Input: part model. Units: mm. Frame: model coordinates. Round coordinates to 2 decimals unless told otherwise and drop trailing zeros. Order: outer loops, then holes, each group sorted by start corner. A loop starts at its lowest first (then second) coordinate and runs counter-clockwise, first axis right, second up. Notation, with made-up numbers: (76, -13) -> (90, -13) arc R34 ccw to (90, 21) -> close; hole circle Ø3 at (14.25, -8.5). An arc over 180 degrees is marked (long way). Use a Markdown table: item, result.
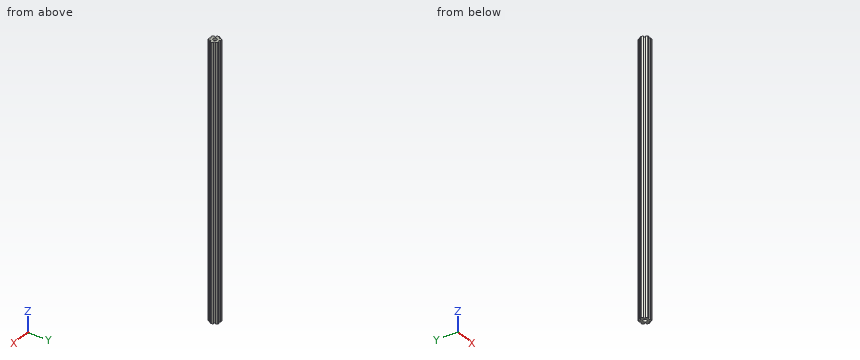
from build123d import *

# Parameters (mm, degrees)
BOSS_EXTRUDE1_DEPTH     = 355.6
SKETCH2_R               = 1.27
SKETCH2_R_2             = 2.54
CUT_EXTRUDE1_DEPTH      = 356.6
FILLET1_R               = 0.508
F_1_4_20_TAPPED_HOLE3_D = 5.1054


with BuildPart() as part:
    # Sketch1 → Boss-Extrude1 (new body)
    with BuildSketch(Plane.XY):
        Polygon((7.332348419, 0), (3.666174209, 6.35), (-3.666174209, 6.35), (-7.332348419, 0), (-3.666174209, -6.35), (3.666174209, -6.35), align=None)
    extrude(amount=BOSS_EXTRUDE1_DEPTH)

    # Sketch2 → Cut-Extrude1 (cut, through all)
    with BuildSketch(Plane.XY.offset(355.6)):
        with Locations((0, 6.35)):
            Circle(SKETCH2_R)
        with Locations((5.499261314, 3.175)):
            Circle(SKETCH2_R)
        with Locations((5.499261314, -3.175)):
            Circle(SKETCH2_R)
        with Locations((0, -6.35)):
            Circle(SKETCH2_R)
        with Locations((-5.499261314, -3.175)):
            Circle(SKETCH2_R)
        with Locations((-5.499261314, 3.175)):
            Circle(SKETCH2_R)
        Circle(SKETCH2_R_2)
    extrude(amount=-CUT_EXTRUDE1_DEPTH, mode=Mode.SUBTRACT)

    # Fillet1
    fillet1_edges = [part.edges().sort_by_distance(p)[0] for p in [
        (3.666174209, -6.35, 177.8),
        (-3.666174209, -6.35, 177.8),
        (-7.332348419, 0, 177.8),
        (-3.666174209, 6.35, 177.8),
        (3.666174209, 6.35, 177.8),
        (7.332348419, 0, 177.8),
    ]]
    fillet(fillet1_edges, radius=FILLET1_R)

    # 1/4-20 Tapped Hole3 (through all)
    with Locations(Plane.XY.offset(355.6)):
        with Locations((0, 0)):
            f_1_4_20_tapped_hole3 = Hole(F_1_4_20_TAPPED_HOLE3_D / 2)

    # Mirror1: 1/4-20 Tapped Hole3 across plane
    add(f_1_4_20_tapped_hole3.mirror(Plane.XY.offset(177.8)), mode=Mode.SUBTRACT)


solid = part.part
1) Contact query for flat-ended pins moving along their axis: P1, Ø1, axis at x = 0, y = -0.5, coming from the +Z side; P2, Ø2, axis at y = -5, z = 223.5, coming from the +X side. Output: stop coordinate, or through.
Answer key:
| item | result |
|---|---|
| P1 | passes through |
| P2 | stops at x = 4.86 |
2) Cut plane A-A on z = 65.5. Return loops of the section in (x, y) (3 decimals), and give its area (3 significant figures).
Answer key:
| item | result |
|---|---|
| outline | (-7.186, -0.254) -> (-6.134, -2.075) arc R1.27 cw to (-4.864, -4.275) -> (-3.813, -6.096) arc R0.508 ccw to (-3.373, -6.35) -> (-1.27, -6.35) arc R1.27 cw to (1.27, -6.35) -> (3.373, -6.35) arc R0.508 ccw to (3.813, -6.096) -> (4.864, -4.275) arc R1.27 cw to (6.134, -2.075) -> (7.186, -0.254) arc R0.508 ccw to (7.186, 0.254) -> (6.134, 2.075) arc R1.27 cw to (4.864, 4.275) -> (3.813, 6.096) arc R0.508 ccw to (3.373, 6.35) -> (1.27, 6.35) arc R1.27 cw to (-1.27, 6.35) -> (-3.373, 6.35) arc R0.508 ccw to (-3.813, 6.096) -> (-4.864, 4.275) arc R1.27 cw to (-6.134, 2.075) -> (-7.186, 0.254) arc R0.508 ccw to start; hole circle Ø5.105 at (0, 0) |
| area | 104 mm^2 |
3) Ray query, probe 1 along Y at (x, z) = (0, 166); probe 2 along Y at (x, z) = (-4.5, 36); probe 3 along X at (y, z) = (-4.25, 39). Return the intervals inside material, ascending.
Answer key:
| item | result |
|---|---|
| probe 1 | y = -5.08 to -2.55, 2.55 to 5.08 |
| probe 2 | y = -4.91 to -3.96, -2.39 to 2.39, 3.96 to 4.91 |
| probe 3 | x = -4.82 to 4.82 |
